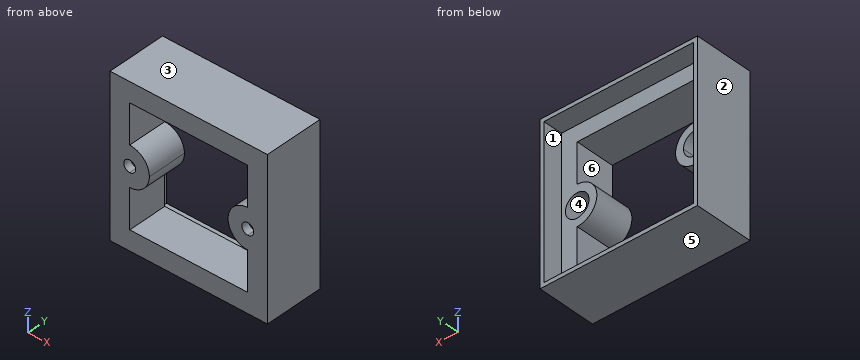
from build123d import *

# Parameters (mm, degrees)
SKETCH1_W           = 40
SKETCH1_H           = 40
SKETCH1_R           = 3
BOSS_EXTRUDE2_DEPTH = 10
BOSS_EXTRUDE3_DEPTH = 10
BOSS_EXTRUDE4_DEPTH = 2
SKETCH2_W           = 40
SKETCH2_H           = 40
SKETCH2_W_2         = 38
SKETCH2_H_2         = 38
BOSS_EXTRUDE5_DEPTH = 5


with BuildPart() as part:
    # Sketch1 → Boss-Extrude2 (new body)
    with BuildSketch(Plane(origin=(0, 0, 0), x_dir=(1, 0, 0), z_dir=(0, 1, 0))):
        Rectangle(SKETCH1_W, SKETCH1_H)
        with BuildLine():
            Line((15, -5), (15, -15))
            Line((15, -15), (-15, -15))
            Line((-15, -15), (-15, -3))
            ThreePointArc((-15, -3), (-18, 0), (-15, 3))
            Line((-15, 3), (-15, 15))
            Line((-15, 15), (15, 15))
            Line((15, 15), (15, 5))
            ThreePointArc((15, 5), (10, 0), (15, -5))
        make_face(mode=Mode.SUBTRACT)
        with Locations(Location((15, 0, 0), (0, 0, 270))):
            Circle(SKETCH1_R, mode=Mode.SUBTRACT)
    extrude(amount=BOSS_EXTRUDE2_DEPTH)

    # Sketch1_4 → Boss-Extrude3 (add)
    with BuildSketch(Plane(origin=(0, 0, 0), x_dir=(1, 0, 0), z_dir=(0, 1, 0))):
        with BuildLine():
            ThreePointArc((-10, 0), (-11.464466094, 3.535533906), (-15, 5))
            Line((-15, 5), (-15, 3))
            ThreePointArc((-15, 3), (-12.878679656, 2.121320344), (-12, 0))
            ThreePointArc((-12, 0), (-12.878679656, -2.121320344), (-15, -3))
            Line((-15, -3), (-15, -5))
            ThreePointArc((-15, -5), (-11.464466094, -3.535533906), (-10, 0))
        make_face()
        with BuildLine():
            Line((-15, 3), (-15, 5))
            ThreePointArc((-15, 5), (-18.535533898, 3.535533914), (-20, 2.3e-08))
            ThreePointArc((-20, 2.3e-08), (-18.535533914, -3.535533898), (-15, -5))
            Line((-15, -5), (-15, -3))
            ThreePointArc((-15, -3), (-18, 0), (-15, 3))
        make_face()
    extrude(amount=BOSS_EXTRUDE3_DEPTH)

    # Sketch1_5 → Boss-Extrude4 (add)
    with BuildSketch(Plane(origin=(0, 0, 0), x_dir=(1, 0, 0), z_dir=(0, 1, 0))):
        with BuildLine():
            ThreePointArc((-12, 0), (-12.878679656, 2.121320344), (-15, 3))
            Line((-15, 3), (-15, 1.5))
            ThreePointArc((-15, 1.5), (-13.939339828, 1.060660172), (-13.5, 0))
            ThreePointArc((-13.5, 0), (-13.939339828, -1.060660172), (-15, -1.5))
            Line((-15, -1.5), (-15, -3))
            ThreePointArc((-15, -3), (-12.878679656, -2.121320344), (-12, 0))
        make_face()
        with BuildLine():
            Line((-15, 1.5), (-15, 3))
            ThreePointArc((-15, 3), (-18, 0), (-15, -3))
            Line((-15, -3), (-15, -1.5))
            ThreePointArc((-15, -1.5), (-16.5, 0), (-15, 1.5))
        make_face()
        with BuildLine():
            ThreePointArc((18, 0), (17.121320344, 2.121320344), (15, 3))
            Line((15, 3), (15, 1.5))
            ThreePointArc((15, 1.5), (16.060660172, 1.060660172), (16.5, 0))
            ThreePointArc((16.5, 0), (16.060660172, -1.060660172), (15, -1.5))
            Line((15, -1.5), (15, -3))
            ThreePointArc((15, -3), (17.121320344, -2.121320344), (18, 0))
        make_face()
        with BuildLine():
            Line((15, 1.5), (15, 3))
            ThreePointArc((15, 3), (12, 0), (15, -3))
            Line((15, -3), (15, -1.5))
            ThreePointArc((15, -1.5), (13.5, 0), (15, 1.5))
        make_face()
    extrude(amount=BOSS_EXTRUDE4_DEPTH)

    # Sketch2 → Boss-Extrude5 (add)
    with BuildSketch(Plane(origin=(0, 10, 0), x_dir=(1, 0, 0), z_dir=(0, 1, 0))):
        Rectangle(SKETCH2_W, SKETCH2_H)
        Rectangle(SKETCH2_W_2, SKETCH2_H_2, mode=Mode.SUBTRACT)
    extrude(amount=BOSS_EXTRUDE5_DEPTH)


solid = part.part
Check sheet for the modelled part. Datum: model origin and axes. Units: mm. Face numbers are marked on the shaded views. A direction names the side the tool comes from. Coordinates: 2 decimals unless noted, no trailing zeros. Write each loop counter-clockwise with the first axis right and the second up, starting at its lowest first coordinate (ties: lowest second). Pieces come first, ordered by that corner, then holes. Notation, with made-up numbers: M 81.5,86 L 98.5,86 A24 cw 98.5,106 Z; hole C 85.5,27.5 d7. An arc over 180 degrees is marked long. Answer as CSV lines item,"result".
Q1. Cross-section at C-C (y = 1.5). Record the boundary of the cut face in (x, z).
Check result:
outline,"M -20,-20 L 20,-20 L 20,20 L -20,20 Z; hole C -15,0 d3; hole M -15,-15 L 15,-15 L 15,-5 A5 cw 15,5 L 15,15 L -15,15 L -15,5 A5 cw -15,-5 Z; hole C 15,0 d3"
Q2. Cross-section at B-B (z = -6). Record the boundary of the cut face in (x, y), then the cut area to 3 significant figures.
Check result:
outline,"M -20,0 L -15,0 L -15,10 L -19,10 L -19,15 L -20,15 Z; M 15,0 L 20,0 L 20,15 L 19,15 L 19,10 L 15,10 Z"
area,"110 mm^2"
Q3. Set-up check for the marked faces 4, 5 and 6: record each of +Z, -Z, +X, -X, +Y, -Y from which the full face is reachable in a straight line by a thin tool's end or side.
Check result:
face 4,"+Y"
face 5,"-Z, +X, -X, +Y, -Y"
face 6,"+Y, -Y"
Q4. Material ranges on probe 1 along X at (y, z) = (6, 0); probe 2 along Z at (x, y) = (-15, 12.25); probe 3 along Z at (x, y) = (1, 6.25), recorded low to high. Write a range as from..to.
Check result:
probe 1,"-20..-18, -12..-10, 10..12, 18..20"
probe 2,"-20..-19, 19..20"
probe 3,"-20..-15, 15..20"
Q5. Cross-section at D-D (x = 14). Record the boundary of the cut face in (y, z).
Check result:
outline,"M 0,-20 L 15,-20 L 15,-19 L 10,-19 L 10,-15 L 0,-15 Z; M 0,-4.9 L 10,-4.9 L 10,-2.83 L 2,-2.83 L 2,-1.12 L 0,-1.12 Z; M 0,1.12 L 2,1.12 L 2,2.83 L 10,2.83 L 10,4.9 L 0,4.9 Z; M 0,15 L 10,15 L 10,19 L 15,19 L 15,20 L 0,20 Z"
Q6. Mould release check, pull along Z, two halves, no side actions. Record for the marked faces 1, 2 and 3: released by +Z, released by -Z, zero draft, split by the parting line, or undercut.
Check result:
face 1,"undercut"
face 2,"zero draft"
face 3,"released by +Z"
Q7. Cross-section at A-A (x = -7). Record the boundary of the cut face in (y, z), then the cut area to 3 significant figures.
Check result:
outline,"M 0,-20 L 15,-20 L 15,-19 L 10,-19 L 10,-15 L 0,-15 Z; M 0,15 L 10,15 L 10,19 L 15,19 L 15,20 L 0,20 Z"
area,"110 mm^2"
Q8. Go/stop test with flat-tipped pins: pin 1 (4 mm diameter, centred on x = -14, z = 13.5, fed in from -Y); pin 2 (5.5 mm diameter, centred on x = 15, z = 0, fed in from +Y). Record where each tip stops, or that it passes through.
Check result:
pin 1,"y = 0"
pin 2,"y = 2"
